from build123d import *

# Parameters (mm, degrees)
F1_DEPTH = 5
F2_W     = 14
F2_H     = 14
F3_DEPTH = 5
F4_R     = 5


with BuildPart() as f1:
    # F0 (on Top) → F1 (new body)
    with BuildSketch(Plane.XY):
        Polygon((0, 15), (0, 0), (0, -15), (100, -15), (254.793411, -23), (254.793411, 0), (254.793411, 23), (100, 15), align=None)
    extrude(amount=F1_DEPTH)

    # F2 (on Top) → F3 (cut, through all)
    with BuildSketch(Plane.XY):
        with Locations((14.239932, 0)):
            Rectangle(F2_W, F2_H)
    extrude(amount=F3_DEPTH, mode=Mode.SUBTRACT)

    # F4
    f4_edges = [f1.edges().sort_by_distance(p)[0] for p in [
        (254.793411, -23, 2.5),
        (254.793411, 23, 2.5),
    ]]
    fillet(f4_edges, radius=F4_R)


solid = f1.part
Could you check a few things on this model? Use its own coordinates, in mm. A direction names the side the tool comes from. Give positions to 0.01 mm unless a question says otherwise; leave off trailing zeros. Order: outer loops, then holes, each group sorted by start corner. A loop starts at its lowest first (then second) coordinate and runs counter-clockwise, first axis right, second up.
1. I need wall thicknesses on L1, parallel to X at y = 2, z = 2.8; L2, parallel to Y at x = 11, z = 2.25; L3, parallel to Y at x = 95, z = 2.05. Which ranges of each line are inside material? Lowest first, please.
Answers below:
L1: x = 0 to 7.24, 21.24 to 254.79
L2: y = -15 to -7, 7 to 15
L3: y = -15 to 15
2. Suppose I cut it at C-C (x = 58.5). Write out the boundary of the cut face in (y, z).
Answers below:
outline: (-15, 0) - (15, 0) - (15, 5) - (-15, 5) - close
3. Suppose I cut it at A-A (y = -2). Write out the boundary of the cut face in (x, z), plus the area to 3 significant figures.
Answers below:
outline: (0, 0) - (7.24, 0) - (7.24, 5) - (0, 5) - close; (21.24, 0) - (254.79, 0) - (254.79, 5) - (21.24, 5) - close
area: 1,200 mm2
4. Suppose I cut it at D-D (y = 20). Write out the boundary of the cut face in (x, z), plus the area to 3 significant figures.
Answers below:
outline: (196.75, 0) - (254.25, 0) - (254.25, 5) - (196.75, 5) - close
area: 288 mm2
5. Thinking about a two-plate mould opening in Y: for faces 4 (the flat face through (51, 15, 2)), 5 (the cylindrical face through (253.195, -21.399, 2.535)), 6 (the flat face through (14, -7, 2)), which applies, +Y half, -Y half, draft (parallel to the pull), parting line (faces both ways), or undercut?
Answers below:
face 4: +Y half
face 5: -Y half
face 6: undercut
6. Which directions (+Z, -Z, +X, -X, +Y, -Y) give clear straight access to the entire face, cutting with the end or side of a thin tool? Please do faces 1 (the flat face through (49, -15, 2)), 2 (the flat face through (7.24, 0, 2)), 3 (the flat face through (175.814, 18.918, 2.465)).
Answers below:
face 1: +Z, -Z, -X, -Y
face 2: +Z, -Z
face 3: +Z, -Z, -X, +Y
7. For pin 1 (1.5 mm diameter, centred on x = 14, z = 1.5, fed in from +Y); pin 2 (1.5 mm diameter, centred on x = 164.5, z = 3, fed in from +Y); pin 3 (1.5 mm diameter, centred on x = 17, z = 2, fed in from -Y), each with a flat end and sliding along its axis, tell me the tip position at first contact or that it passes through.
Answers below:
pin 1: stops at y = 15
pin 2: stops at y = 18.37
pin 3: stops at y = -15
8. Suppose I cut it at B-B (z = 3.15). Write out the boundary of the cut face in (x, y), plus the area to 3 significant figures.
Answers below:
outline: (0, -15) - (100, -15) - (249.54, -22.73) arc R5 ccw to (254.79, -17.73) - (254.79, 17.73) arc R5 ccw to (249.54, 22.73) - (100, 15) - (0, 15) - close; hole (7.24, -7) - (21.24, -7) - (21.24, 7) - (7.24, 7) - close
area: 8,670 mm2
